For this review, use the dimensioned drawing (mm, ordinates from the lowest corner) and the shaded views. A direction names the side the tool comes from. Give positions to 0.01 mm unless a question says otherwise; leave off trailing zeros. Loops run counter-clockwise (first coordinate to the right, second up) from the corner with the lowest first, then second, coordinate; pieces in that order, holes last. Notation, with made-up numbers: (71.5, 23) - (105.5, 23) arc R7 ccw to (105.5, 33) - close; hole circle Ø6 at (-38.5, 68.25). An arc over 180 degrees is marked (long way). Write each question's results on one line, items separated by ' | '.
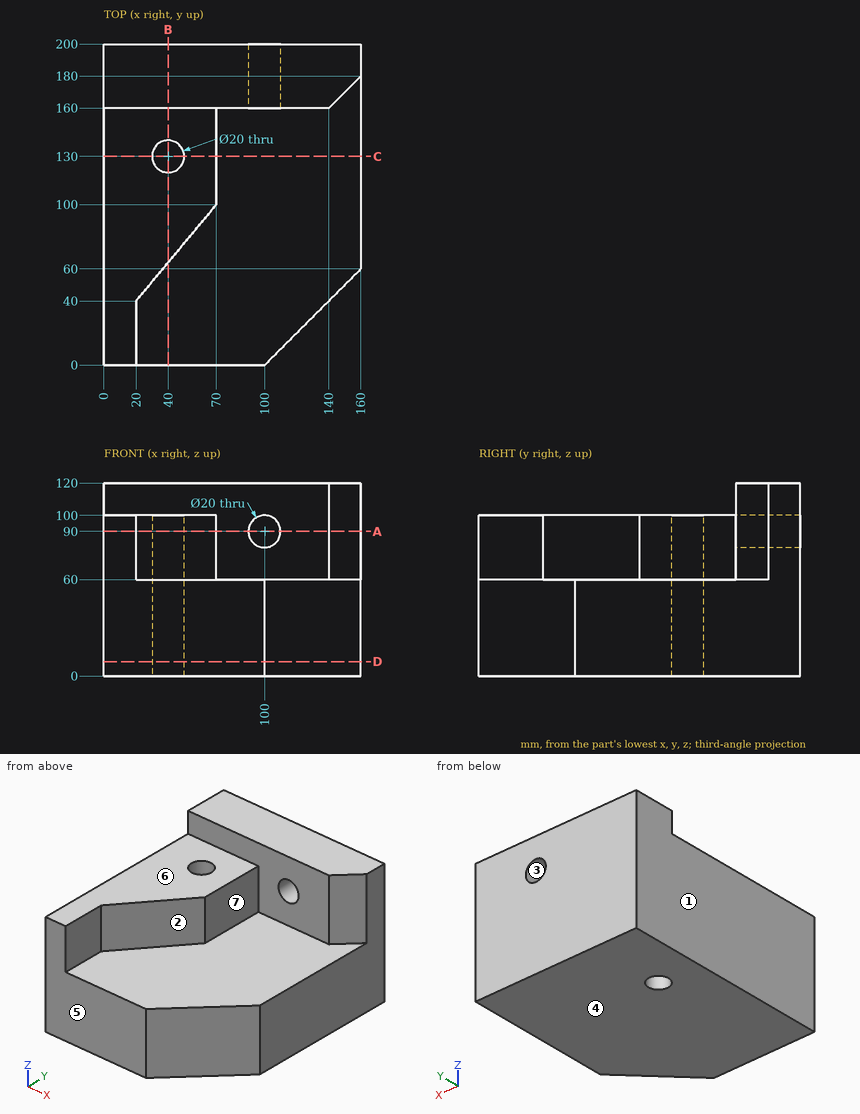
Item 1: We need section D-D on z = 9. Give the boundary of the cut face in (x, y), then the cut area to 3 significant figures.
Output values:
outline: (0, 0) - (100, 0) - (160, 60) - (160, 200) - (0, 200) - close; hole circle Ø20 at (40, 130) | area: 29,900 mm²
Item 2: We need section C-C on y = 130. Give the boundary of the cut face in (x, z).
Output values:
outline: (0, 0) - (30, 0) - (30, 100) - (0, 100) - close; (50, 0) - (160, 0) - (160, 60) - (70, 60) - (70, 100) - (50, 100) - close
Item 3: Clearance check with flat-ended pins moving along their axes: P1, Ø5, axis at x = 70.5, z = 70.5, coming from the -Y side; P2, Ø16, axis at x = 40, y = 130, coming from the +Z side; P3, Ø10, axis at y = 152, z = 89, coming from the +X side; P4, Ø5, axis at x = 52, y = 83, coming from the +Z side. State where each tip first meets the part, or that it passes through.
Output values:
P1: stops at y = 97.6 | P2: passes through | P3: stops at x = 70 | P4: stops at z = 100
Item 4: Wall thickness on probe 1 along Z at (x, y) = (100, 179.5); probe 2 along X at (y, z) = (130, 40.5); probe 3 along Z at (x, y) = (63, 13): over which ranges is each line inside the solid? List them lowest first.
Output values:
probe 1: z = 0 to 80, 100 to 120 | probe 2: x = 0 to 30, 50 to 160 | probe 3: z = 0 to 60
Item 5: We need section B-B on x = 40. Give the boundary of the cut face in (y, z).
Output values:
outline: (0, 0) - (120, 0) - (120, 100) - (64, 100) - (64, 60) - (0, 60) - close; (140, 0) - (200, 0) - (200, 120) - (160, 120) - (160, 100) - (140, 100) - close
Item 6: We need section A-A on z = 90. Give the boundary of the cut face in (x, y).
Output values:
outline: (0, 0) - (20, 0) - (20, 40) - (70, 100) - (70, 160) - (90, 160) - (90, 200) - (0, 200) - close; (110, 160) - (140, 160) - (160, 180) - (160, 200) - (110, 200) - close; hole circle Ø20 at (40, 130)
Item 7: Tool access review of the marked faces 5, 6 and 7: name each direction out of +Z, -Z, +X, -X, +Y, -Y from which nothing blocks a thin tool from reaching the whole face with its end or side.
Output values:
face 5: +Z, -Z, +X, -X, -Y | face 6: +Z, +X, -X, -Y | face 7: +Z, +X, -Y
Item 8: Draft analysis for pull direction X (two halves, no side actions). For the marked faces 1, 2, 3 and 4, state which applies: +X half, -X half, draft (parallel to the pull), parting line (faces both ways), or undercut.
Output values:
face 1: -X half | face 2: +X half | face 3: undercut | face 4: draft
